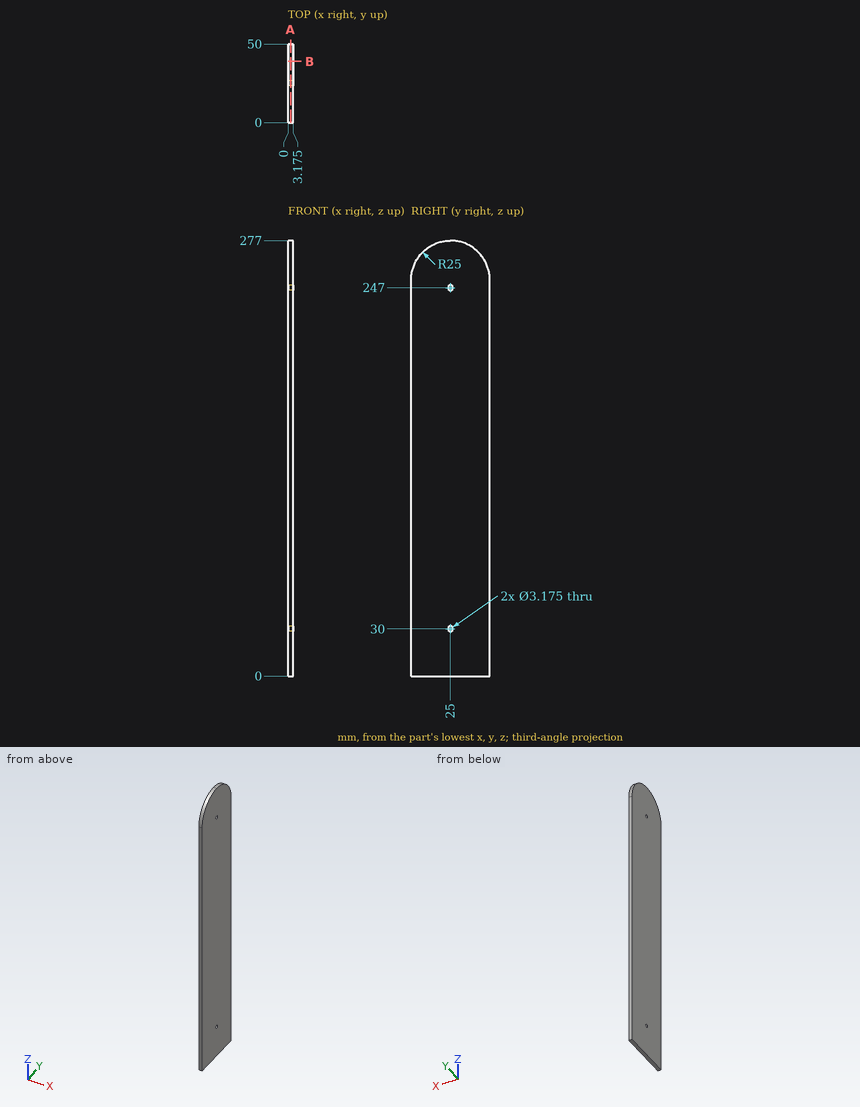
Drawing for the job (mm, zero at the part's lowest x, y, z). Give positions to 0.01 mm unless a question says otherwise; leave off trailing zeros. Order: outer loops, then holes, each group sorted by start corner. A loop starts at its lowest first (then second) coordinate and runs counter-clockwise, first axis right, second up. Notation, with made-up numbers: M 34.25,25 L 78.25,25 A27 ccw 78.25,56 Z; hole C 40.25,68 d2. An arc over 180 degrees is marked long. Use a Markdown table: item, result. Add a question column.
(1) Probe line 1 along Z through (x, y) = (2.5, 25); line 2 along Z through (x, y) = (3.05, 25.5) (3 decimals); line 3 along Y through (x, z) = (2.15, 247). List the from-to ranges inside material, lowest first. Write a range as [from, to].
(2) Saw through at A-A, the plane x = 1.6. Give the number of separate pieces and of enclosed holes in the cut face, and give its area (3 significant figures).
(3) Saw through at B-B, the plane y = 39. Give the cut face in (x, z) (3 decimals).
Answer key:
| question | item | result |
|---|---|---|
| 1 | line 1 | [0, 28.41], [31.59, 245.41], [248.59, 277] |
| 1 | line 2 | [0, 28.493], [31.507, 245.493], [248.507, 276.995] |
| 1 | line 3 | [0, 23.41], [26.59, 50] |
| 2 | separate pieces | 1 |
| 2 | enclosed holes | 2 |
| 2 | area | 13,600 mm^2 |
| 3 | outline | M 0,0 L 3.175,0 L 3.175,272.712 L 0,272.712 Z |
